from build123d import *

# Parameters (mm, degrees)
SKETCH1_W           = 20
SKETCH1_H           = 40
BOSS_EXTRUDE1_DEPTH = 15
SKETCH2_W           = 20
SKETCH2_H           = 20
BOSS_EXTRUDE2_DEPTH = 10
BOSS_EXTRUDE3_DEPTH = 5
BOSS_EXTRUDE4_DEPTH = 5
BOSS_EXTRUDE5_DEPTH = 5
BOSS_EXTRUDE6_DEPTH = 15
SKETCH7_R           = 2.1
SKETCH7_R_2         = 2
CUT_EXTRUDE1_DEPTH  = 108.703296143
FILLET5_R           = 1
SKETCH9_W           = 40
SKETCH9_H           = 15
CUT_EXTRUDE2_DEPTH  = 20


with BuildPart() as part:
    # Sketch1 → Boss-Extrude1 (new body)
    with BuildSketch(Plane(origin=(0, 0, 0), x_dir=(1, 0, 0), z_dir=(0, 1, 0))):
        with Locations((10, -20)):
            Rectangle(SKETCH1_W, SKETCH1_H)
    extrude(amount=BOSS_EXTRUDE1_DEPTH)

    # Sketch2 → Boss-Extrude2 (add)
    with BuildSketch(Plane(origin=(0, 15, 0), x_dir=(1, 0, 0), z_dir=(0, 1, 0))):
        with Locations((10, -20)):
            Rectangle(SKETCH2_W, SKETCH2_H)
    extrude(amount=BOSS_EXTRUDE2_DEPTH)

    # Sketch3 → Boss-Extrude3 (add)
    with BuildSketch(Plane.XY.offset(27.5)):
        with BuildLine():
            Line((10, 35), (10, 25))
            Line((10, 25), (0, 25))
            Line((0, 25), (0, 31.846606339))
            ThreePointArc((0, 31.846606339), (-17.534478591, 63.08453427), (10, 86))
            Line((10, 86), (10, 81))
            ThreePointArc((10, 81), (-13, 58), (10, 35))
        make_face()
    extrude(amount=-BOSS_EXTRUDE3_DEPTH)

    # Sketch4 → Boss-Extrude4 (add)
    with BuildSketch(Plane(origin=(0, 0, 22.5), x_dir=(-1, 0, 0), z_dir=(0, 0, -1))):
        with BuildLine():
            Line((-10, 86), (-10, 84))
            ThreePointArc((-10, 84), (16, 58), (-10, 32))
            Line((-10, 32), (-10, 30))
            Line((-10, 30), (-10, 25))
            Line((-10, 25), (0, 25))
            Line((0, 25), (0, 31.846606339))
            ThreePointArc((0, 31.846606339), (17.534478591, 63.08453427), (-10, 86))
        make_face()
    extrude(amount=BOSS_EXTRUDE4_DEPTH)

    # Sketch5 → Boss-Extrude5 (add)
    with BuildSketch(Plane(origin=(0, 0, 17.5), x_dir=(-1, 0, 0), z_dir=(0, 0, -1))):
        with BuildLine():
            Line((-10, 86), (-10, 81))
            ThreePointArc((-10, 81), (13, 58), (-10, 35))
            Line((-10, 35), (-10, 30))
            Line((-10, 30), (-10, 25))
            Line((-10, 25), (0, 25))
            Line((0, 25), (0, 31.846606339))
            ThreePointArc((0, 31.846606339), (17.534478591, 63.08453427), (-10, 86))
        make_face()
    extrude(amount=BOSS_EXTRUDE5_DEPTH)

    # Sketch6 → Boss-Extrude6 (add)
    with BuildSketch(Plane.XY.offset(27.5)):
        with BuildLine():
            Line((10, 86), (10, 96))
            Line((10, 96), (2.753066737, 96))
            Line((2.753066737, 96), (2.753066737, 85.045923136))
            ThreePointArc((2.753066737, 85.045923136), (6.345266618, 85.760456118), (10, 86))
        make_face()
    extrude(amount=-BOSS_EXTRUDE6_DEPTH)

    # Sketch7 → Cut-Extrude1 (cut, through all)
    with BuildSketch(Plane(origin=(10, 0, 0), x_dir=(0, 0, -1), z_dir=(1, 0, 0))):
        with Locations((-20, 91)):
            Circle(SKETCH7_R)
        with Locations((-20, 28.5)):
            Circle(SKETCH7_R_2)
    extrude(amount=-CUT_EXTRUDE1_DEPTH, mode=Mode.SUBTRACT)

    # Fillet5
    fillet5_edges = [part.edges().sort_by_distance(p)[0] for p in [
        (10, 82.5, 22.5),
        (-13, 58, 22.5),
        (10, 81, 25),
        (10, 35, 25),
        (-13, 58, 27.5),
        (10, 33.5, 22.5),
        (-16, 58, 22.5),
        (10, 84, 20),
        (10, 32, 20),
        (-16, 58, 17.5),
        (10, 82.5, 17.5),
        (-13, 58, 17.5),
        (10, 81, 15),
        (10, 33.5, 17.5),
        (10, 35, 15),
        (-13, 58, 12.5),
    ]]
    fillet(fillet5_edges, radius=FILLET5_R)

    # Sketch9 → Cut-Extrude2 (cut)
    with BuildSketch(Plane(origin=(20, 0, 0), x_dir=(0, 0, -1), z_dir=(1, 0, 0))):
        with Locations((-20, 7.5)):
            Rectangle(SKETCH9_W, SKETCH9_H)
    extrude(amount=-CUT_EXTRUDE2_DEPTH, mode=Mode.SUBTRACT)


solid = part.part
Build history of the part. All positions in model axes, mm. A direction names the side the tool comes from. Give positions to 0.01 mm unless a question says otherwise; leave off trailing zeros. Order: outer loops, then holes, each group sorted by start corner. A loop starts at its lowest first (then second) coordinate and runs counter-clockwise, first axis right, second up. Notation, with made-up numbers: M 77.5,36.25 L 110.5,36.25 A12 cw 110.5,50.25 Z; hole C 70,54.25 d2. An arc over 180 degrees is marked long. Put each result on its own line as item: value.
Item 1: Cut at C-C on z = 15.25. Write the cut outline in (x, y), then the cut area to 3 significant figures.
Results are:
outline: M 0,15 L 20,15 L 20,25 L 10,25 L 10,34.02 A1 ccw 9.04,35.02 A23 cw 9.04,80.98 A1 ccw 10,81.98 L 10,96 L 2.75,96 L 2.75,85.05 A28 ccw 0,31.85 Z
area: 731 mm2
Item 2: Wall check: probe 1 along Y at (x, z) = (2, 20); probe 2 along Y at (x, z) = (3, 18.25); probe 3 along Y at (x, z) = (5, 20). Give the ranges that are in metal, low to high.
Results are:
probe 1: 15 to 26.5, 30.5 to 33.26, 82.74 to 84.83
probe 2: 15 to 27.53, 29.47 to 32.99, 83.01 to 89.84, 92.16 to 96
probe 3: 15 to 26.5, 30.5 to 32.49, 83.51 to 88.9, 93.1 to 96
Item 3: Drop flat-ended pins along their axis: pin 1 Ø1.5 at (y, z) = (66.5, 20.5) entering from -X; pin 2 Ø12 at (y, z) = (49, 15.5) entering from -X; pin 3 Ø1.5 at (y, z) = (69, 26) entering from +X. Give the stop position or say it passes through.
Results are:
pin 1: x = -16.91
pin 2: x = -17.84
pin 3: x = -9.77
Item 4: Cut at A-A on z = 20. Write the cut outline in (x, y), then the cut area to 3 significant figures.
Results are:
outline: M 0,15 L 20,15 L 20,25 L 10,25 L 10,26.5 L 0,26.5 Z; M 0,30.5 L 10,30.5 L 10,31.02 A1 ccw 9.04,32.02 A26 cw 9.04,83.98 A1 ccw 10,84.98 L 10,88.9 L 2.75,88.9 L 2.75,85.05 A28 ccw 0,31.85 Z; M 2.75,93.1 L 10,93.1 L 10,96 L 2.75,96 Z
area: 430 mm2
Item 5: Cut at B-B on y = 91. Write the cut outline in (x, z).
Results are:
outline: M 2.75,12.5 L 10,12.5 L 10,17.9 L 2.75,17.9 Z; M 2.75,22.1 L 10,22.1 L 10,27.5 L 2.75,27.5 Z
Item 6: Which spindle directions (+Z, -Z, +X, -X, +Y, -Y) get a long thin tool onto all of the face, cutting with end or side? Do faces 1 (the face through (10, 89, 22)), 2 (the face through (-14, 61, 12.5)), 3 (the face through (-14, 61, 27.5)), 4 (the face through (-14.5, 58.1, 17.5)). Say none if no direction does.
Results are:
face 1: +Z, -Z, +X, +Y
face 2: -Z, +X, -X, +Y
face 3: +Z, +X, -X, +Y
face 4: +X
Item 7: Cut at D-D on y = 58. Write the cut outline in (x, z), then the cut area to 3 significant figures.
Results are:
outline: M -18,12.5 L -14,12.5 A1 ccw -13,13.5 L -13,16.5 A1 ccw -14,17.5 L -15,17.5 A1 cw -16,18.5 L -16,21.5 A1 cw -15,22.5 L -14,22.5 A1 ccw -13,23.5 L -13,26.5 A1 ccw -14,27.5 L -18,27.5 Z
area: 59.6 mm2
Item 8: Pull direction Y, two halves, no side cores. Call faces 5 (the face through (-17.984, 58.955, 20.105)), 6 (the face through (-15.994, 58.558, 20.021)), 7 (the face through (14, 25, 20)): +Y half, -Y half, draft (parallel to the pull), parting line (faces both ways), or undercut.
Results are:
face 5: parting line
face 6: undercut
face 7: +Y half
